Here's how the part is built. I have some questions about the finished solid (model axes, mm). Face numbers are marked on the shaded views. Coordinates: 2 decimals unless noted, no trailing zeros. Loops run counter-clockwise (first coordinate to the right, second up) from the corner with the lowest first, then second, coordinate; pieces in that order, holes last.
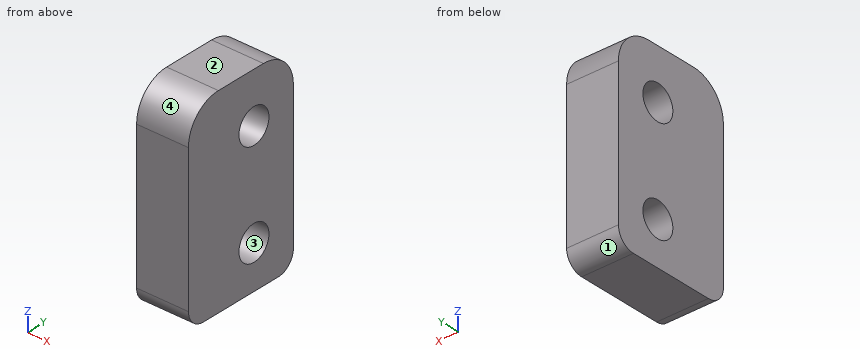
from build123d import *

# Parameters (mm, degrees)
SKETCH1_R           = 1
BOSS_EXTRUDE1_DEPTH = 3
FILLET1_R           = 2
FILLET2_R           = 1


with BuildPart() as part:
    # Sketch1 → Boss-Extrude1 (new body)
    with BuildSketch(Plane(origin=(0, 0, 0), x_dir=(0, 0, -1), z_dir=(1, 0, 0))):
        Polygon((-1.868695944, 2.63), (2.5, 2.63), (2.5, -4.37), (-8.91, -4.37), (-8.91, 2.63), align=None)
        Circle(SKETCH1_R, mode=Mode.SUBTRACT)
        with Locations((-6, 0)):
            Circle(SKETCH1_R, mode=Mode.SUBTRACT)
    extrude(amount=-BOSS_EXTRUDE1_DEPTH)

    # Fillet1
    fillet1_edges = [part.edges().sort_by_distance(p)[0] for p in [
        (-1.5, -4.37, 8.91),
        (-1.5, 2.63, 8.91),
    ]]
    fillet(fillet1_edges, radius=FILLET1_R)

    # Fillet2
    fillet2_edges = [part.edges().sort_by_distance(p)[0] for p in [
        (-1.5, 2.63, -2.5),
        (-1.5, -4.37, -2.5),
    ]]
    fillet(fillet2_edges, radius=FILLET2_R)


solid = part.part
Q1. Suppose I cut it at B-B on z = 6. Write out the boundary of the cut face in (x, y), and give its area (3 significant figures).
Q2. Suppose I cut it at D-D on y = 0.75. Write out the boundary of the cut face in (x, z).
Q3. Suppose I cut it at A-A on y = 0. Write out the boundary of the cut face in (x, z), and give its area (3 significant figures).
Q4. Suppose I cut it at C-C on x = -1.9. Write out the boundary of the cut face in (y, z), and give its area (3 significant figures).
Q5. Please list where these lines run through material, in increasing order: probe 1 along Z at (x, y) = (-2.8, 0.25); probe 2 along Y at (x, z) = (-1.4, 6); probe 3 along Z at (x, y) = (-0.35, 0.5).
Q6. We'd pull the mould along Y, two halves only. Please class the marked faces 1, 2, 3 and 4: pulls with the +Y half, pulls with the -Y half, needs draft (parallel to the pull), parting line crosses it, or undercut.
Check values:
1. outline: (-3, -4.37) - (0, -4.37) - (0, -1) - (-3, -1) - close; (-3, 1) - (0, 1) - (0, 2.63) - (-3, 2.63) - close
1. area: 15.0 mm2
2. outline: (-3, -2.5) - (0, -2.5) - (0, -0.66) - (-3, -0.66) - close; (-3, 0.66) - (0, 0.66) - (0, 5.34) - (-3, 5.34) - close; (-3, 6.66) - (0, 6.66) - (0, 8.91) - (-3, 8.91) - close
3. outline: (-3, -2.5) - (0, -2.5) - (0, -1) - (-3, -1) - close; (-3, 1) - (0, 1) - (0, 5) - (-3, 5) - close; (-3, 7) - (0, 7) - (0, 8.91) - (-3, 8.91) - close
3. area: 22.2 mm2
4. outline: (-4.37, -1.5) arc R1 ccw to (-3.37, -2.5) - (1.63, -2.5) arc R1 ccw to (2.63, -1.5) - (2.63, 6.91) arc R2 ccw to (0.63, 8.91) - (-2.37, 8.91) arc R2 ccw to (-4.37, 6.91) - close; hole circle Ø2 at (0, 0); hole circle Ø2 at (0, 6)
4. area: 71.4 mm2
5. probe 1: z = -2.5 to -0.97, 0.97 to 5.03, 6.97 to 8.91
5. probe 2: y = -4.37 to -1, 1 to 2.63
5. probe 3: z = -2.5 to -0.87, 0.87 to 5.13, 6.87 to 8.91
6. face 1: pulls with the +Y half
6. face 2: needs draft
6. face 3: undercut
6. face 4: pulls with the -Y half
